Could you check a few things on this drawing? It's one solid part, dimensions in mm from its lowest x, y, z. Give positions to 0.01 mm unless a question says otherwise; leave off trailing zeros. Loops run counter-clockwise (first coordinate to the right, second up) from the corner with the lowest first, then second, coordinate; pieces in that order, holes last.
1. I need wall thicknesses on line 1 along X through (y, z) = (67, 0.4); line 2 along Y through (x, z) = (67.5, 1.6). Which ranges of each line are inside material? Lowest first, please.
2. Imagine slicing it at A-A (x = 22.5). List the corners of the cut face in (y, z) for me.
3. Imagine slicing it at B-B (z = 1.1). Count the separate pieces of the cut face and the enclosed holes in it, plus the area to 3 significant figures.
4. Imagine slicing it at C-C (y = 67.5). List the corners of the cut face in (x, z) for me, plus the area to 3 significant figures.
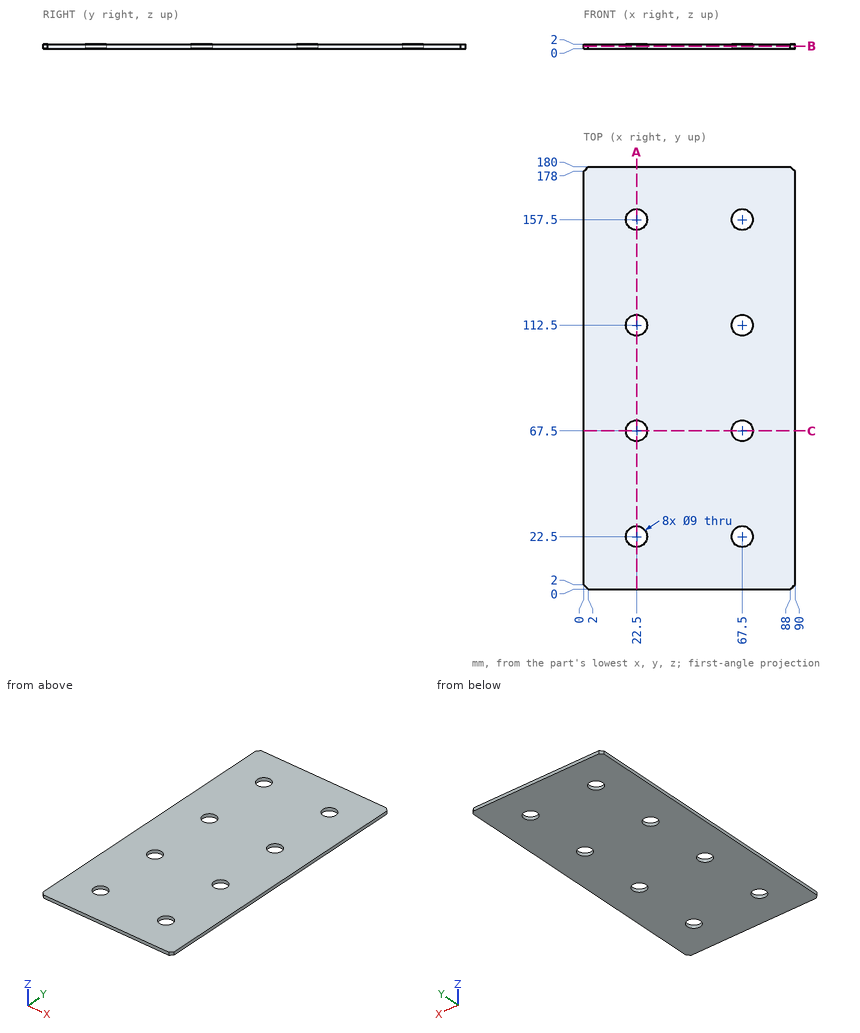
Derived:
1. line 1: x = 0 to 18.03, 26.97 to 63.03, 71.97 to 90
1. line 2: y = 0 to 18, 27 to 63, 72 to 108, 117 to 153, 162 to 180
2. outline: (0, 0) - (18, 0) - (18, 2) - (0, 2) - close; (27, 0) - (63, 0) - (63, 2) - (27, 2) - close; (72, 0) - (108, 0) - (108, 2) - (72, 2) - close; (117, 0) - (153, 0) - (153, 2) - (117, 2) - close; (162, 0) - (180, 0) - (180, 2) - (162, 2) - close
3. separate pieces: 1
3. enclosed holes: 8
3. area: 15,700 mm2
4. outline: (0, 0) - (18, 0) - (18, 2) - (0, 2) - close; (27, 0) - (63, 0) - (63, 2) - (27, 2) - close; (72, 0) - (90, 0) - (90, 2) - (72, 2) - close
4. area: 144 mm2
